```python
from build123d import *

# Parameters (mm, degrees)
F0_W      = 80
F0_H      = 280
F1_DEPTH  = 15
F3_DEPTH  = 80
F4_W      = 11
F4_H      = 22
F5_DEPTH  = 15
F7_R      = 3
F7_R_2    = 6.556779
F8_DEPTH  = 280.001
F9_R      = 3
F10_DEPTH = 80.001


with BuildPart() as f1:
    # F0 (on Top) → F1 (new body)
    with BuildSketch(Plane.XY):
        with Locations((40, 140)):
            Rectangle(F0_W, F0_H)
    extrude(amount=F1_DEPTH)

    # F2 (on face) → F3 (join)
    with BuildSketch(Plane.YZ.offset(80)):
        Polygon((65.358984, 35), (60, 15), (82.717968, 15), (77.358984, 35), align=None)
    extrude(amount=-F3_DEPTH)

    # F4 (on face) → F5 (cut, through all)
    with BuildSketch(Plane.XY.offset(15)):
        with Locations((5.5, 14)):
            Rectangle(F4_W, F4_H)
    extrude(amount=-F5_DEPTH, mode=Mode.SUBTRACT)

    # F7 (on face) → F8 (cut, through all)
    with BuildSketch(Plane.XZ):
        with Locations((60, 6)):
            Circle(F7_R)
        with Locations((-491.183044, 5.330358)):
            Circle(F7_R_2)
        with Locations((20, 6)):
            Circle(F7_R)
    extrude(amount=-F8_DEPTH, mode=Mode.SUBTRACT)

    # F9 (on face) → F10 (cut, through all)
    with BuildSketch(Plane.YZ.offset(80)):
        with Locations((50, 6)):
            Circle(F9_R)
        with Locations((150, 6)):
            Circle(F9_R)
        with Locations((250, 6)):
            Circle(F9_R)
    extrude(amount=-F10_DEPTH, mode=Mode.SUBTRACT)


solid = f1.part
```
CAD build for the part. Positions are in the model's coordinates, mm. A direction names the side the tool comes from. Round coordinates to 2 decimals unless told otherwise and drop trailing zeros. Loops run counter-clockwise (first coordinate to the right, second up) from the corner with the lowest first, then second, coordinate; pieces in that order, holes last. Notation, with made-up numbers: M 47,60.25 L 85,60.25 A26 cw 85,78.25 Z; hole C 22,2 d8. An arc over 180 degrees is marked long. Use a Markdown table: item, result. Add a question column.
(1) Drill centre lines: line 1 (Y direction, x = 73.5, z = 6); line 2 (Z direction, x = 71, y = 150); line 3 (Y direction, x = 8, z = 10.5). Where is each one in solid material? Low to high.
(2) Flat gauge pins, fed straight in: pin 1 (3.5 mm diameter, centred on y = 150, z = 6, fed in from +X); pin 2 (12 mm diameter, centred on x = 63, z = 30, fed in from -Y); pin 3 (10 mm diameter, centred on x = 28, y = 212.5, fed in from +Z); pin 4 (12 mm diameter, centred on y = 17, z = 7, fed in from -X). Where does each tip first touch, or does it go through?
(3) Cut at B-B (y = 143). Give the cut face in (x, z).
(4) Cut at C-C (z = 6). State how many separate pieces and enclosed holes the cut face has, and give its area (3 significant figures).
(5) Cut at A-A (x = 73). Give the cut face in (y, z), and give its area (3 significant figures).
(6) Cut at D-D (y = 68). Give the cut face in (x, z).
(7) Pull direction Z, two halves, no side cores. Call faces 4 (the face through (17.6, 24.6, 4.2)), 5 (the face through (39, 30, 15)), 6 (the face through (0, 151, 9)): +Z half, -Z half, draft (parallel to the pull), parting line (faces both ways), or undercut.
(8) Which spindle directions (+Z, -Z, +X, -X, +Y, -Y) get a long thin tool onto all of the face, cutting with end or side? Do faces 1 (the face through (5, 25, 8)), 2 (the face through (39, 183, 15)), 3 (the face through (40.56, 62.717, 25.14)). Say none if no direction does.
Geometry says:
| question | item | result |
|---|---|---|
| 1 | line 1 | y = 0 to 47, 53 to 147, 153 to 247, 253 to 280 |
| 1 | line 2 | z = 0 to 3, 9 to 15 |
| 1 | line 3 | y = 0 to 3, 25 to 280 |
| 2 | pin 1 | passes through |
| 2 | pin 2 | stops at y = 62.41 |
| 2 | pin 3 | stops at z = 15 |
| 2 | pin 4 | stops at x = 11 |
| 3 | outline | M 0,0 L 80,0 L 80,15 L 0,15 Z; hole C 20,6 d6; hole C 60,6 d6 |
| 4 | separate pieces | 12 |
| 4 | enclosed holes | 0 |
| 4 | area | 17,600 mm² |
| 5 | outline | M 0,0 L 280,0 L 280,15 L 82.72,15 L 77.36,35 L 65.36,35 L 60,15 L 0,15 Z; hole C 50,6 d6; hole C 150,6 d6; hole C 250,6 d6 |
| 5 | area | 4,460 mm² |
| 6 | outline | M 0,0 L 80,0 L 80,35 L 0,35 Z; hole C 20,6 d6; hole C 60,6 d6 |
| 7 | face 4 | undercut |
| 7 | face 5 | +Z half |
| 7 | face 6 | draft |
| 8 | face 1 | +Z, -Z, -X |
| 8 | face 2 | +Z, +X, -X, +Y |
| 8 | face 3 | +Z, +X, -X, -Y |
